Print and shaded views of the part. All mm, measured from the part's lowest x, y and z. A direction names the side the tool comes from. Give positions to 0.01 mm unless a question says otherwise; leave off trailing zeros. Write each loop counter-clockwise with the first axis right and the second up, starting at its lowest first coordinate (ties: lowest second). Pieces come first, ordered by that corner, then holes. Notation, with made-up numbers: (36, 43.5) -> (78, 43.5) arc R12 cw to (78, 48.5) -> close; hole circle Ø5 at (2, 29.5). An arc over 180 degrees is marked (long way). Put each result on its own line as item: value.
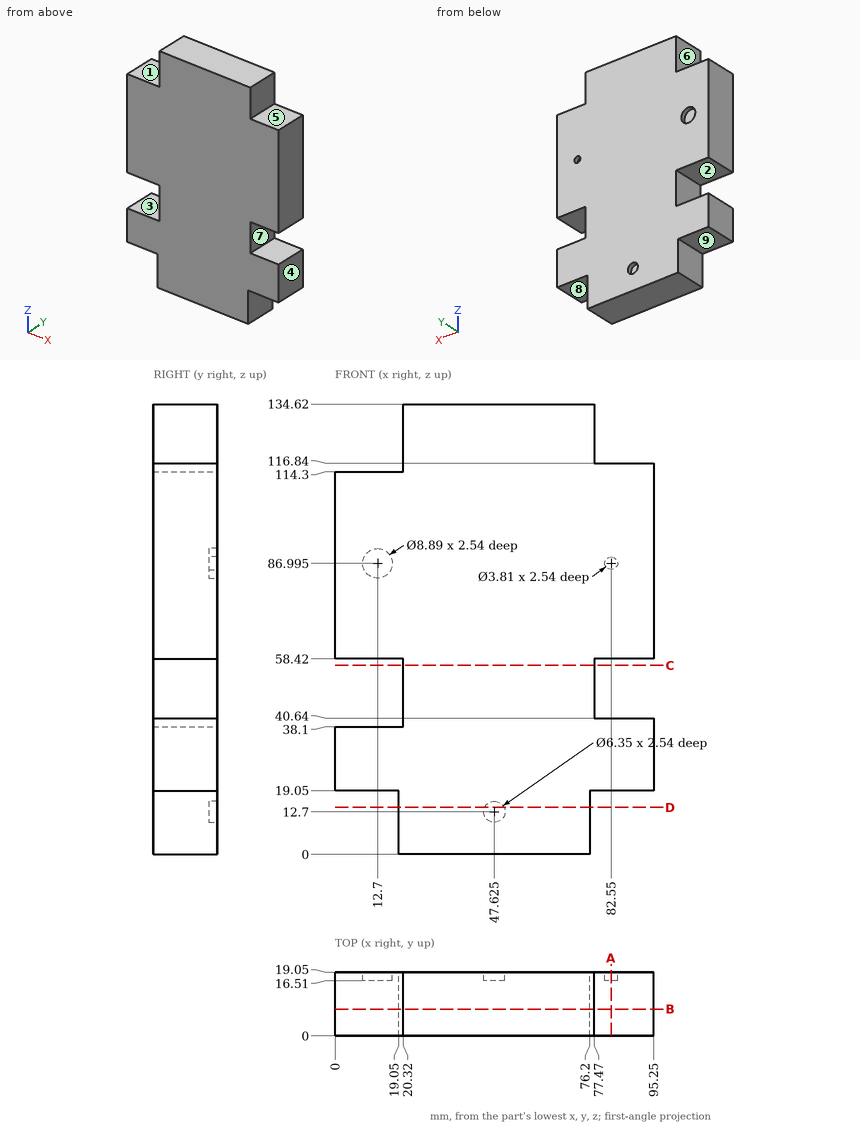
1) Slice it at D-D (z = 14). Write the cut outline in (x, y), plus the area to 3 significant figures.
Filled sheet:
outline: (19.05, 0) -> (76.2, 0) -> (76.2, 19.05) -> (50.52, 19.05) -> (50.52, 16.51) -> (44.73, 16.51) -> (44.73, 19.05) -> (19.05, 19.05) -> close
area: 1,070 mm2
2) Slice it at C-C (z = 56.5). Write the cut outline in (x, y), plus the area to 3 significant figures.
Filled sheet:
outline: (20.32, 0) -> (77.47, 0) -> (77.47, 19.05) -> (20.32, 19.05) -> close
area: 1,090 mm2
3) Tool access for the marked faces 5, 6, 7, 8 and 9: list every direction of +Z, -Z, +X, -X, +Y, -Y with a clear straight run to the whole face (end or side of a thin tool).
Filled sheet:
face 5: +Z, +X, +Y, -Y
face 6: +Z, -X, +Y, -Y
face 7: +X, +Y, -Y
face 8: -Z, +X, +Y, -Y
face 9: -Z, -X, +Y, -Y
4) Slice it at A-A (x = 82.55). Write the cut outline in (y, z), plus the area to 3 significant figures.
Filled sheet:
outline: (0, 19.05) -> (19.05, 19.05) -> (19.05, 40.64) -> (0, 40.64) -> close; (0, 58.42) -> (19.05, 58.42) -> (19.05, 85.09) -> (16.51, 85.09) -> (16.51, 88.9) -> (19.05, 88.9) -> (19.05, 116.84) -> (0, 116.84) -> close
area: 1,510 mm2
5) Slice it at B-B (y = 8). Write the cut outline in (x, z), plus the area to 3 significant figures.
Filled sheet:
outline: (0, 19.05) -> (19.05, 19.05) -> (19.05, 0) -> (76.2, 0) -> (76.2, 19.05) -> (95.25, 19.05) -> (95.25, 40.64) -> (77.47, 40.64) -> (77.47, 58.42) -> (95.25, 58.42) -> (95.25, 116.84) -> (77.47, 116.84) -> (77.47, 134.62) -> (20.32, 134.62) -> (20.32, 114.3) -> (0, 114.3) -> (0, 58.42) -> (20.32, 58.42) -> (20.32, 38.1) -> (0, 38.1) -> close
area: 10,600 mm2
6) Pull direction Z, two halves, no side cores. Call the marked faces 1, 2, 3 and 4: released by +Z, released by -Z, zero draft, split by the parting line, or undercut.
Filled sheet:
face 1: released by +Z
face 2: undercut
face 3: undercut
face 4: zero draft
7) Pin check, flat tips, straight feed: pin 1 (9.5 mm diameter, centred on x = 87, y = 11, fed in from -Z); pin 2 (1.9 mm diameter, centred on x = 82, z = 87, fed in from +Y); pin 3 (2 mm diameter, centred on y = 8, z = 17.5, fed in from +X). Stop position of each tip, or through.
Filled sheet:
pin 1: z = 19.05
pin 2: y = 16.51
pin 3: x = 76.2
8) Wall check: L1, parallel to Z at x = 82.55, y = 18.35; L2, parallel to Z at x = 19, y = 7.75; L3, parallel to X at y = 18.1, z = 12.7. Give the ranges that are in metal, low to high.
Filled sheet:
L1: 19.05 to 40.64, 58.42 to 85.09, 88.9 to 116.84
L2: 19.05 to 38.1, 58.42 to 114.3
L3: 19.05 to 44.45, 50.8 to 76.2
